Source: CAD feature listing. Evaluate the final solid. Frame: model axes, mm. A direction names the side the tool comes from. Round coordinates to 2 decimals unless told otherwise and drop trailing zeros. Order: outer loops, then holes, each group sorted by start corner. A loop starts at its lowest first (then second) coordinate and runs counter-clockwise, first axis right, second up. Notation, with made-up numbers: (-24.75, 6) -> (6.25, 6) arc R17 ccw to (6.25, 10) -> close; hole circle Ø3 at (67, 67). An arc over 180 degrees is marked (long way). Write item = value, one per line. Start each with the question number.
(1) Ray query, line 1 (Y direction, x = 0, z = -320) (3 decimals); line 2 (Z direction, x = -9, y = 18); line 3 (Z direction, x = -19, y = 3.5) (3 decimals). Return the intervals inside material, ascending.
(2) Contact query for flat-ended pins moving along their axis: pin 1 Ø2.5 at (y, z) = (11, -285) entering from +X; pin 2 Ø1.5 at (y, z) = (-12.5, -38) entering from +X; pin 3 Ø4 at (x, z) = (-9.5, -114.5) entering from -Y; pin 4 Ø10 at (x, y) = (-0.5, -1) entering from -Z. Output: stop coordinate, or through.
(3) Cut plane A-A on z = -156. Return the cut outline in (x, y).
(4) Cut plane C-C on z = -280.5. Return the cut outline in (x, y), then the cut area to 3 significant figures.
(5) Draft query along X for faces 1 (the face through (0, 10, -274)), 2 (the face through (-7, 19, -141)), 3 (the face through (-4.44, 4.07, -316.07)), 4 (the face through (-19.98, -0.88, -198.03)). Return one class per face: released by +X, released by -X, zero draft, split by the parting line, or undercut.
(6) Reachability of faces 5 (the face through (8.06, -12.65, -52.18)), 6 (the face through (2.44, 18.59, -186.86)), 7 (the face through (5, 5, -331)), 8 (the face through (0, 0, 0)), 9 (the face through (-1.82, -13.88, -270.32)) from +Z, -Z, +X, -X, +Y, -Y: full face, straight path, thin tool, end or side. Return the list, or none.
(7) Cut plane B-B on z = -23. Return the cut outline in (x, y).
from build123d import *

# Parameters (mm, degrees)
CHAMFER_1_SIZE         = 3
HOLE_WIZARD_M121_D     = 10.2
HOLE_WIZARD_M121_DEPTH = 30
HOLE_WIZARD_M121_TIP   = 3.064389157
SKETCH_4_R             = 20
SKETCH_4_R_2           = 18.75
CUT_EXTRUDE_1_DEPTH    = 1.85
FILLET_1_R             = 0.05
CHAMFER_2_SIZE         = 1.5
CUT_EXTRUDE_2_DEPTH    = 334.782863551
SKETCH_9_R             = 25
SKETCH_9_R_2           = 20
CUT_EXTRUDE_4_DEPTH    = 6
CHAMFER_3_SIZE         = 1.5
CHAMFER_4_SIZE         = 3


# Read off the part's stored shape, not the designer's step: Условная геометрия резьбовых отверстий
with BuildPart() as part:
    # Эскиз1 → Повернуть1 (revolve)
    with BuildSketch(Plane(origin=(0, 0, 0), x_dir=(0, 0, -1), z_dir=(1, 0, 0)), mode=Mode.PRIVATE) as revolve_1_sk:
        Polygon((0, 0), (0, 15), (100, 15), (100, 25), (147, 25), (147, 20), (211, 20), (211, 14), (331, 14), (331, 0), align=None)
    revolve(revolve_1_sk.sketch.rotate(Axis((0, 0, 0), (0, 0, -1)), 90), axis=Axis((0, 0, 0), (0, 0, -1)))

    # Фаска1
    chamfer_1_edges = [part.edges().sort_by_distance(p)[0] for p in [
        (-25, 0, -100),
        (-15, 0, 0),
        (-14, 0, -331),
    ]]
    chamfer(chamfer_1_edges, length=CHAMFER_1_SIZE)

    # Отверстие обработанное метчиком M121
    with Locations(Plane(origin=(0, 0, -331), x_dir=(-1, 0, 0), z_dir=(0, 0, -1))):
        with Locations((0, 0)):
            Hole(HOLE_WIZARD_M121_D / 2, depth=HOLE_WIZARD_M121_DEPTH)
            with Locations((0, 0, -(HOLE_WIZARD_M121_DEPTH + HOLE_WIZARD_M121_TIP / 2))):  # 118° drill point
                Cone(0, HOLE_WIZARD_M121_D / 2, HOLE_WIZARD_M121_TIP, mode=Mode.SUBTRACT)

    # Эскиз4 → Вырез-Вытянуть1 (cut)
    with BuildSketch(Plane(origin=(0, 0, -187.775), x_dir=(-1, 0, 0), z_dir=(0, 0, -1))):
        with Locations(Location((0, 0, 0), (0, 0, 180))):
            Circle(SKETCH_4_R)
        Circle(SKETCH_4_R_2, mode=Mode.SUBTRACT)
    extrude(amount=-CUT_EXTRUDE_1_DEPTH, mode=Mode.SUBTRACT)

    # Скругление1
    fillet_1_edges = [part.edges().sort_by_distance(p)[0] for p in [
        (18.75, 0, -185.925),
        (18.75, 0, -187.775),
    ]]
    fillet(fillet_1_edges, radius=FILLET_1_R)

    # Фаска2
    chamfer_2_edges = [part.edges().sort_by_distance(p)[0] for p in [
        (-25, 0, -147),
    ]]
    chamfer(chamfer_2_edges, length=CHAMFER_2_SIZE)

    # Эскиз8 → Вырез-Вытянуть2 (cut, through all)
    with BuildSketch(Plane(origin=(0, 10, -331), x_dir=(-1, 0, 0), z_dir=(0, -1, 0))):
        with BuildLine():
            Line((4, -30), (4, -85))
            ThreePointArc((4, -85), (0, -89), (-4, -85))
            Line((-4, -85), (-4, -30))
            ThreePointArc((-4, -30), (0, -26), (4, -30))
        make_face()
    extrude(amount=-CUT_EXTRUDE_2_DEPTH, mode=Mode.SUBTRACT)

    # Эскиз9 → Вырез-Вытянуть4 (cut)
    with BuildSketch(Plane(origin=(0, 0, -147), x_dir=(-1, 0, 0), z_dir=(0, 0, -1))):
        Circle(SKETCH_9_R)
        Circle(SKETCH_9_R_2, mode=Mode.SUBTRACT)
    extrude(amount=-CUT_EXTRUDE_4_DEPTH, mode=Mode.SUBTRACT)

    # Фаска3
    chamfer_3_edges = [part.edges().sort_by_distance(p)[0] for p in [
        (-25, 0, -141),
    ]]
    chamfer(chamfer_3_edges, length=CHAMFER_3_SIZE)

    # Фаска4
    chamfer_4_edges = [part.edges().sort_by_distance(p)[0] for p in [
        (-20, 0, -211),
    ]]
    chamfer(chamfer_4_edges, length=CHAMFER_4_SIZE)

    # Move Face 2213 outline → Move Face 2213 (revolve, cut)
    with BuildSketch(Plane.XZ):
        Polygon((6.025, -301.555796073), (5.1, -301), (5.1, -331), (6.025, -331), align=None)
    revolve(axis=Axis((0, 0, 0), (0, 0, 1)), mode=Mode.SUBTRACT)


solid = part.part
Evaluation:
q1.line_1 = -14 to -6.025, 6.025 to 14
q1.line_2 = -141 to -100
q1.line_3 = -208.68 to -187.775, -185.925 to -100
q2.pin_1 = 10.05
q2.pin_2 = 9.32
q2.pin_3 = -23.85
q2.pin_4 = -331
q3.outline = circle Ø40 at (0, 0)
q4.outline = (-4, 10) -> (-4, 13.42) arc R14 ccw (long way) to (4, 13.42) -> (4, 10) -> close
q4.area = 585 mm^2
q5.face_1 = undercut
q5.face_2 = zero draft
q5.face_3 = undercut
q5.face_4 = split by the parting line
q6.face_5 = +Z
q6.face_6 = none
q6.face_7 = -Z, +X, -X, +Y, -Y
q6.face_8 = +Z, +X, -X, +Y, -Y
q6.face_9 = -Z
q7.outline = circle Ø30 at (0, 0)
